Read the model definition and answer for the solid it produces. Units are mm, in the model's axes. Face numbers are marked on the shaded views. A direction names the side the tool comes from. Round coordinates to 2 decimals unless told otherwise and drop trailing zeros. Order: outer loops, then holes, each group sorted by start corner. A loop starts at its lowest first (then second) coordinate and runs counter-clockwise, first axis right, second up.
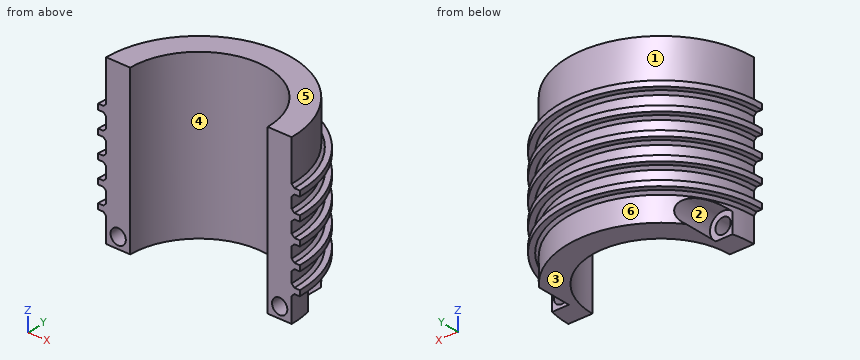
Autodesk Inventor part; units mm, degrees
ref_plane "Work Plane1" through (0, 0, 27.94) normal (0, 0, 1) x (1, 0, 0)
ref_plane "Work Plane2" through (16.002, 25.4, 0) normal (0, -1, 0) x (1, 0, 0)
ref_plane "YZ Plane" through (0, 0, 0) normal (1, 0, 0) x (0, 1, 0)
sketch "Sketch1" plane through (0, 0, 0) normal (0, 0, 1) x (1, 0, 0)
  arc A0 (16.002, 0) -> (-16.002, 0) centre (0, 0) ccw
  arc A1 (21.59, 0) -> (-21.59, 0) centre (0, 0) ccw
  line L0 (-16.002, 0) -> (-21.59, 0)
  line L1 (16.002, 0) -> (21.59, 0)
  dimension "d0" = 43.18
  dimension "d1" = 32.004
extrude "Extrusion1" add sketch "Sketch1" along normal blind 38.1
ref_plane "Work Plane1" through (0, 0, 27.94) normal (0, 0, 1) x (1, 0, 0)
sketch "Sketch2" plane through (0, 0, 27.94) normal (0, 0, 1) x (1, 0, 0)
  arc A0 (21.59, 0) -> (-21.59, 0) centre (0, 0) ccw
  arc A1 (23.495, 0) -> (-23.495, 0) centre (0, 0) ccw
  line L0 (-21.59, 0) -> (-23.495, 0)
  line L1 (16.002, 0) -> (21.59, 0)
  line L2 (23.495, 0) -> (21.59, 0)
  dimension "d5" = 1.905
extrude "Extrusion2" add sketch "Sketch2" against normal blind 1.27
chamfer "Chamfer1" distance 0.635 angle 45 2 edges at (0, 21.59, 27.94) (0, 21.59, 26.67)
pattern_linear "Rectangular Pattern1" count 5 spacing 5.08 along (0, 0, -1) of "Extrusion2", "Chamfer1"
sketch "Sketch3" plane through (16.002, 0, 0) normal (0, -1, 0) x (1, 0, 0)
  line L0 (0, 0) -> (5.588, 0) construction
  line L1 (5.588, 0) -> (5.588, 5.715) construction
  line L2 (6.223, 6.35) -> (5.588, 5.715) construction
  line L3 (7.493, 6.35) -> (6.223, 6.35) construction
  line L4 (7.493, 7.62) -> (7.493, 6.35) construction
  line L5 (7.493, 7.62) -> (6.223, 7.62) construction
  line L6 (5.588, 8.255) -> (6.223, 7.62) construction
  line L7 (5.588, 8.255) -> (5.588, 10.795) construction
  line L8 (6.223, 11.43) -> (5.588, 10.795) construction
  line L9 (7.493, 11.43) -> (6.223, 11.43) construction
  line L10 (7.493, 12.7) -> (7.493, 11.43) construction
  line L11 (7.493, 12.7) -> (6.223, 12.7) construction
  line L12 (5.588, 13.335) -> (6.223, 12.7) construction
  line L13 (5.588, 13.335) -> (5.588, 15.875) construction
  line L14 (6.223, 16.51) -> (5.588, 15.875) construction
  line L15 (7.493, 16.51) -> (6.223, 16.51) construction
  line L16 (7.493, 17.78) -> (7.493, 16.51) construction
  line L17 (7.493, 17.78) -> (6.223, 17.78) construction
  line L18 (5.588, 18.415) -> (6.223, 17.78) construction
  line L19 (5.588, 18.415) -> (5.588, 20.955) construction
  line L20 (6.223, 21.59) -> (5.588, 20.955) construction
  line L21 (7.493, 21.59) -> (6.223, 21.59) construction
  line L22 (7.493, 22.86) -> (7.493, 21.59) construction
  line L23 (7.493, 22.86) -> (6.223, 22.86) construction
  line L24 (5.588, 23.495) -> (6.223, 22.86) construction
  line L25 (5.588, 23.495) -> (5.588, 26.035) construction
  line L26 (6.223, 26.67) -> (5.588, 26.035) construction
  line L27 (7.493, 26.67) -> (6.223, 26.67) construction
  line L28 (7.493, 27.94) -> (7.493, 26.67) construction
  line L29 (7.493, 27.94) -> (6.223, 27.94) construction
  line L30 (5.588, 28.575) -> (6.223, 27.94) construction
  line L31 (5.588, 28.575) -> (5.588, 38.1) construction
  line L32 (0, 38.1) -> (5.588, 38.1) construction
  line L33 (0, 0) -> (0, 38.1) construction
  line L34 (-37.592, 0) -> (-32.004, 0) construction
  line L35 (-32.004, 0) -> (-32.004, 38.1) construction
  line L36 (-37.592, 38.1) -> (-32.004, 38.1) construction
  line L37 (-37.592, 28.575) -> (-37.592, 38.1) construction
  line L38 (-38.227, 27.94) -> (-37.592, 28.575) construction
  line L39 (-38.227, 27.94) -> (-39.497, 27.94) construction
  line L40 (-39.497, 27.94) -> (-39.497, 26.67) construction
  line L41 (-38.227, 26.67) -> (-39.497, 26.67) construction
  line L42 (-37.592, 26.035) -> (-38.227, 26.67) construction
  line L43 (-37.592, 23.495) -> (-37.592, 26.035) construction
  line L44 (-38.227, 22.86) -> (-37.592, 23.495) construction
  line L45 (-38.227, 22.86) -> (-39.497, 22.86) construction
  line L46 (-39.497, 22.86) -> (-39.497, 21.59) construction
  line L47 (-38.227, 21.59) -> (-39.497, 21.59) construction
  line L48 (-37.592, 20.955) -> (-38.227, 21.59) construction
  line L49 (-37.592, 18.415) -> (-37.592, 20.955) construction
  line L50 (-38.227, 17.78) -> (-37.592, 18.415) construction
  line L51 (-38.227, 17.78) -> (-39.497, 17.78) construction
  line L52 (-39.497, 17.78) -> (-39.497, 16.51) construction
  line L53 (-38.227, 16.51) -> (-39.497, 16.51) construction
  line L54 (-37.592, 15.875) -> (-38.227, 16.51) construction
  line L55 (-37.592, 13.335) -> (-37.592, 15.875) construction
  line L56 (-38.227, 12.7) -> (-37.592, 13.335) construction
  line L57 (-38.227, 12.7) -> (-39.497, 12.7) construction
  line L58 (-39.497, 12.7) -> (-39.497, 11.43) construction
  line L59 (-38.227, 11.43) -> (-39.497, 11.43) construction
  line L60 (-37.592, 10.795) -> (-38.227, 11.43) construction
  line L61 (-37.592, 8.255) -> (-37.592, 10.795) construction
  line L62 (-38.227, 7.62) -> (-37.592, 8.255) construction
  line L63 (-38.227, 7.62) -> (-39.497, 7.62) construction
  line L64 (-39.497, 7.62) -> (-39.497, 6.35) construction
  line L65 (-38.227, 6.35) -> (-39.497, 6.35) construction
  line L66 (-37.592, 5.715) -> (-38.227, 6.35) construction
  line L67 (-37.592, 0) -> (-37.592, 5.715) construction
  circle A0 centre (2.794, 2.54) radius 1.778
  circle A1 centre (-34.798, 2.54) radius 1.778
  point P0 (-16.002, 0)
  dimension "d14" = 3.556
  dimension "d15" = 2.54
  dimension "d16" = 3.556
extrude "Extrusion3" cut sketch "Sketch3" against normal through all
ref_plane "Work Plane2" through (16.002, 25.4, 0) normal (0, -1, 0) x (1, 0, 0)
sketch "Sketch4" plane through (16.002, 25.4, 0) normal (0, -1, 0) x (1, 0, 0)
  circle A0 centre (2.794, 2.54) radius 1.778 construction
  circle A1 centre (-34.798, 2.54) radius 1.778 construction
  circle A2 centre (2.794, 2.54) radius 3.048
  circle A3 centre (-34.798, 2.54) radius 3.048
  line L0 (2.794, -0.508) -> (7.3935, -0.1769)
  line L1 (7.3935, -0.1769) -> (6.0075, 2.6942)
  line L2 (6.0075, 2.6942) -> (5.8411, 2.6139)
  line L3 (-34.7976, -0.508) -> (-34.7976, -3.1659)
  line L4 (-34.7976, -3.1659) -> (-38.8338, -2.6207)
  line L5 (-38.8338, -2.6207) -> (-39.8503, 2.0729)
  line L6 (-39.8503, 2.0729) -> (-37.8451, 2.6139)
  point P0 (-16.002, 0)
  dimension "d20" = 6.096
  dimension "d21" = 6.096
extrude "Extrusion4" cut sketch "Sketch4" along normal blind 20.32
properties part number "CoreOpposite" material "ABS Plastic"
Q1. A cutting plane is placed at C-C, the plane z = 25.5. Give the vertices of the cut face in (x, y).
Outcome:
outline: (-21.59, 0) - (-16, 0) arc R16 cw to (16, 0) - (21.59, 0) arc R21.59 ccw to start
Q2. For the marked faces 1, 2 and 3, determine the directions among +Z, -Z, +X, -X, +Y, -Y from which every point of the face is accessible in a straight line to the end or side of a thin tool.
Outcome:
face 1: +Z, +Y
face 2: +Y
face 3: -Z, +X, -X, +Y, -Y
Q3. Straight lines are drawn through the part: probe 1 along Z at (x, y) = (17.5, 14.75); probe 2 along Z at (x, y) = (-11.5, 18.75); probe 3 along X at (y, z) = (12.25, 35). For each, find the intervals that lie inside material, in ascending order.
Outcome:
probe 1: z = 6.35 to 7.62, 11.43 to 12.7, 16.51 to 17.78, 21.59 to 22.86, 26.67 to 27.94
probe 2: z = 6.12 to 7.85, 11.2 to 12.93, 16.28 to 18.01, 21.36 to 23.09, 26.44 to 28.17
probe 3: x = -17.78 to -10.3, 10.3 to 17.78
Q4. A cutting plane is placed at A-A, the plane z = 2.54. Give the vertices of the cut face in (x, y), plus the area to 3 significant figures.
Outcome:
outline: (-21.59, 0) - (-20.57, 0) - (-20.57, 5.08) - (-20.98, 5.08) arc R21.59 ccw to start; (-17.02, 0) - (-16, 0) arc R16 cw to (16, 0) - (17.02, 0) - (17.02, 5.08) - (15.75, 5.08) - (15.75, 14.77) arc R21.59 ccw to (-15.75, 14.77) - (-15.75, 5.08) - (-17.02, 5.08) - close; (20.57, 0) - (21.59, 0) arc R21.59 ccw to (20.98, 5.08) - (20.57, 5.08) - close
area: 233 mm2
Q5. Flat-ended cylindrical pins translate along their axes: pin 1 (5 mm diameter, centred on x = 18.5, z = 13, fed in from +Y); pin 2 (6 mm diameter, centred on x = -18.5, z = 2.5, fed in from +Y); pin 3 (8 mm diameter, centred on y = 19, z = 32, fed in from -X). Find the tip coordinate at first contact, or state that the pin passes through.
Outcome:
pin 1: stops at y = 17.19
pin 2: stops at y = 15.03
pin 3: stops at x = -15.53
Q6. A cutting plane is placed at D-D, the plane y = 3. Give the number of separate pieces and of enclosed holes in the cut face, plus the area to 3 significant figures.
Outcome:
separate pieces: 2
enclosed holes: 2
area: 440 mm2
Q7. For a pull along X with two mould halves and no side action, classify the marked faces 4, 5 and 6 as released by +X, released by -X, zero draft, split by the parting line, or undercut.
Outcome:
face 4: undercut
face 5: zero draft
face 6: split by the parting line
